Check sheet for the drawn part. Datum: minimum x, y, z corner. Units: mm. Give positions to 0.01 mm unless a question says otherwise; leave off trailing zeros. Loops run counter-clockwise (first coordinate to the right, second up) from the corner with the lowest first, then second, coordinate; pieces in that order, holes last. Notation, with made-up numbers: (-4.75, 81.5) - (29.25, 81.5) arc R22 ccw to (29.25, 117.5) - close; hole circle Ø4 at (19.5, 13.25). An arc over 180 degrees is marked (long way). One line per item, written item: value. Start each with the question number.
1. Scan lines: L1, parallel to Y at x = 30, z = 4; L2, parallel to X at y = 96.5, z = 6; L3, parallel to Y at x = 144, z = 7.5. Record each from-to range of solid material in increasing order. Write a range as [from, to].
2. Sectioned sample at D-D (x = 31). Record the cut outline in (y, z).
3. Sectioned sample at B-B (y = 315). Record the cut outline in (x, z).
4. Gauge pin test, flat end, axial feed: pin 1 (20 mm diameter, centred on x = 30, y = 105, fed in from -Z). Record the tip position at first contact, or that the pin passes through.
5. Sectioned sample at A-A (z = 1.5). Count the separate pieces of the cut face and the enclosed holes in it, plus the area to 3 significant figures.
6. Sectioned sample at C-C (x = 150). Record the cut outline in (y, z), plus the area to 3 significant figures.
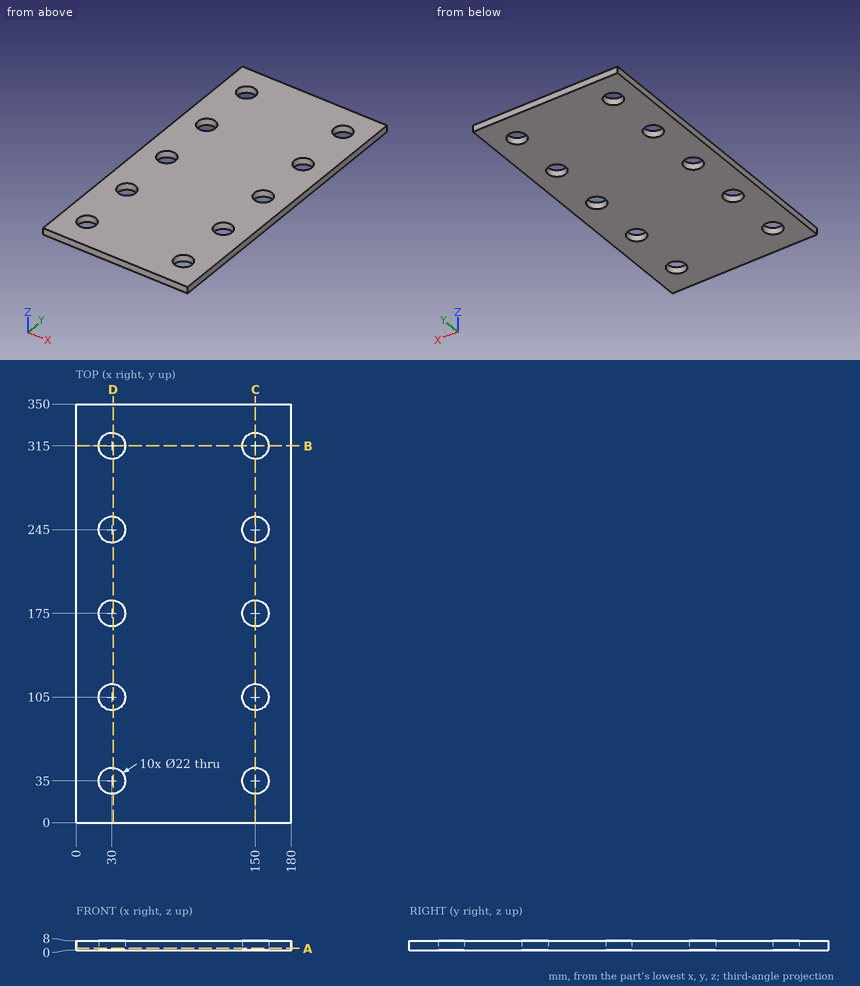
Results are:
1. L1: y = [0, 24], [46, 94], [116, 164], [186, 234], [256, 304], [326, 350]
1. L2: x = [0, 23.02], [36.98, 143.02], [156.98, 180]
1. L3: y = [0, 25.78], [44.22, 95.78], [114.22, 165.78], [184.22, 235.78], [254.22, 305.78], [324.22, 350]
2. outline: (0, 0) - (24.05, 0) - (24.05, 8) - (0, 8) - close; (45.95, 0) - (94.05, 0) - (94.05, 8) - (45.95, 8) - close; (115.95, 0) - (164.05, 0) - (164.05, 8) - (115.95, 8) - close; (185.95, 0) - (234.05, 0) - (234.05, 8) - (185.95, 8) - close; (255.95, 0) - (304.05, 0) - (304.05, 8) - (255.95, 8) - close; (325.95, 0) - (350, 0) - (350, 8) - (325.95, 8) - close
3. outline: (0, 0) - (19, 0) - (19, 8) - (0, 8) - close; (41, 0) - (139, 0) - (139, 8) - (41, 8) - close; (161, 0) - (180, 0) - (180, 8) - (161, 8) - close
4. pin 1: passes through
5. separate pieces: 1
5. enclosed holes: 10
5. area: 59,200 mm^2
6. outline: (0, 0) - (24, 0) - (24, 8) - (0, 8) - close; (46, 0) - (94, 0) - (94, 8) - (46, 8) - close; (116, 0) - (164, 0) - (164, 8) - (116, 8) - close; (186, 0) - (234, 0) - (234, 8) - (186, 8) - close; (256, 0) - (304, 0) - (304, 8) - (256, 8) - close; (326, 0) - (350, 0) - (350, 8) - (326, 8) - close
6. area: 1,920 mm^2
